Work out the finished part from the listing and answer in its coordinate system (mm). A direction names the side the tool comes from. Coordinates: 2 decimals unless noted, no trailing zeros. Order: outer loops, then holes, each group sorted by start corner. A loop starts at its lowest first (then second) coordinate and runs counter-clockwise, first axis right, second up. Notation, with made-up numbers: (-28.75, 17) -> (-24.75, 17) arc R32 cw to (-24.75, 50) -> close; hole circle Ø7 at (-11, -26.75). An arc over 180 degrees is marked (long way). Use one line per item in the form item = value.
from build123d import *

# Parameters (mm, degrees)
SKETCH1_R                       = 20
BOSS_EXTRUDE1_DEPTH             = 74
SKETCH2_R                       = 2.5
BOSS_EXTRUDE2_DEPTH             = 20
BOSS_EXTRUDE2_DIRECTION_2_REACH = 76
CUT_EXTRUDE1_DEPTH              = 3.81
SKETCH7_R                       = 1.526021313
CUT_EXTRUDE2_DEPTH              = 8.89


with BuildPart() as part:
    # Sketch1 → Boss-Extrude1 (new body)
    with BuildSketch(Plane(origin=(0, 0, 0), x_dir=(0, 0, -1), z_dir=(1, 0, 0))):
        Circle(SKETCH1_R)
    extrude(amount=BOSS_EXTRUDE1_DEPTH)

    # Sketch5 → Cut-Revolve1 (revolve, cut)
    with BuildSketch(Plane(origin=(0, 0, 0), x_dir=(1, 0, 0), z_dir=(0, 1, 0))):
        Polygon((0, 19.337777094), (0.662222906, 20), (0.662222906, 20.176229402), (4.550138216, 20.176229402), (4.550138216, 19.930023338), (4.572872876, 19.930023338), (4.572872876, 20.70759824), (0.489891522, 20.70759824), (-0.879929624, 19.337777094), align=None)
        Polygon((0, 0), (0.645058213, 0), (0.645058213, 3.416287186), (0.081805863, 3.416287186), (0, 3.498093049), (-0.347704824, 3.498093049), (-0.347704824, 0), align=None)
    revolve(axis=Axis((-44.161448521, 0, 0), (1, 0, 0)), mode=Mode.SUBTRACT)

    # Sketch2 → Boss-Extrude2 (add)
    with BuildSketch(Plane.ZY):
        Circle(SKETCH2_R)
    extrude(amount=BOSS_EXTRUDE2_DEPTH)

    # Sketch2 → Boss-Extrude2 direction 2 (add, up to next)
    with BuildSketch(Plane.ZY, mode=Mode.PRIVATE) as boss_extrude2_direction_2_sk1:
        Circle(SKETCH2_R)
    boss_extrude2_direction_2_tool1 = extrude(boss_extrude2_direction_2_sk1.sketch, amount=-BOSS_EXTRUDE2_DIRECTION_2_REACH, mode=Mode.PRIVATE) - part.part
    add(boss_extrude2_direction_2_tool1.solids().sort_by_distance((0, 0, 0))[0])

    # Sketch6 → Cut-Extrude1 (cut)
    with BuildSketch(Plane.ZY):
        with BuildLine():
            Line((-2.93474373, 16.742014233), (-2.93474373, 20.766805635))
            Line((-2.93474373, 20.766805635), (2.93474373, 20.766805635))
            Line((2.93474373, 20.766805635), (2.93474373, 16.742014233))
            ThreePointArc((2.93474373, 16.742014233), (0, 13.807270503), (-2.93474373, 16.742014233))
        make_face()
        with BuildLine():
            Line((20.766805635, -2.93474373), (16.742014233, -2.93474373))
            ThreePointArc((16.742014233, -2.93474373), (13.807270503, 0), (16.742014233, 2.93474373))
            Line((16.742014233, 2.93474373), (20.766805635, 2.93474373))
            Line((20.766805635, 2.93474373), (20.766805635, -2.93474373))
        make_face()
        with BuildLine():
            Line((-2.93474373, -20.766805635), (-2.93474373, -16.742014233))
            ThreePointArc((-2.93474373, -16.742014233), (0, -13.807270503), (2.93474373, -16.742014233))
            Line((2.93474373, -16.742014233), (2.93474373, -20.766805635))
            Line((2.93474373, -20.766805635), (-2.93474373, -20.766805635))
        make_face()
        with BuildLine():
            Line((-20.766805635, 2.93474373), (-16.742014233, 2.93474373))
            ThreePointArc((-16.742014233, 2.93474373), (-13.807270503, 0), (-16.742014233, -2.93474373))
            Line((-16.742014233, -2.93474373), (-20.766805635, -2.93474373))
            Line((-20.766805635, -2.93474373), (-20.766805635, 2.93474373))
        make_face()
    extrude(amount=-CUT_EXTRUDE1_DEPTH, mode=Mode.SUBTRACT)

    # Sketch7 → Cut-Extrude2 (cut)
    with BuildSketch(Plane.ZY):
        with Locations((-3.398071731, 12.681776348)):
            Circle(SKETCH7_R)
        with Locations((9.283704617, 9.283704617)):
            Circle(SKETCH7_R)
        with Locations((12.681776348, -3.398071731)):
            Circle(SKETCH7_R)
        with Locations((3.398071731, -12.681776348)):
            Circle(SKETCH7_R)
        with Locations((-9.283704617, -9.283704617)):
            Circle(SKETCH7_R)
        with Locations((-12.681776348, 3.398071731)):
            Circle(SKETCH7_R)
    extrude(amount=-CUT_EXTRUDE2_DEPTH, mode=Mode.SUBTRACT)


solid = part.part
(1) Which of the six approach directions +Z, -Z, +X, -X, +Y, -Y give full straight-line access (tool end or side, diameter ignored) to faces 1 (the flat face through (2, -2.935, -18)), 2 (the flat face through (2, -2.935, 18)), 3 (the cylindrical face through (4.38, -9.22, -10.81)), 4 (the flat face through (2, -18, -2.935))?
Data:
face_1 = -Z, -X
face_2 = +Z, -X
face_3 = -X
face_4 = -X, -Y
(2) Straight lines are drawn through the part: line 1 along Y through (x, z) = (0.4, 0); line 2 along Z through (x, y) = (20.5, -3); line 3 along X through (y, z) = (-12, 4). For each, find the intervals that lie inside material, in ascending order.
Data:
line_1 = -13.81 to -3.42, -2.5 to 2.5, 3.42 to 13.81
line_2 = -19.77 to 19.77
line_3 = 8.89 to 74
(3) Section C-C on x = 50.5 is taken. Write down the section's boundary in (y, z), plus the area to 3 significant figures.
Data:
outline = circle Ø40 at (0, 0)
area = 1,260 mm²
(4) Each of these flat-tipped pins is pushed along its axis until it touches: P1, Ø1, axis at x = 62, y = 6.5, coming from the -Z side; P2, Ø1.5, axis at x = 50.5, y = -4.5, coming from the -Z side; P3, Ø6, axis at x = 51, y = -2.5, coming from the -Z side; P4, Ø10, axis at y = 9, z = 9.5, coming from the -X side. Where does it stop, or does it pass through?
Data:
P1 = -19.08
P2 = -19.65
P3 = -20
P4 = 0
(5) The mould has two halves that part along Y. Classify faces 5 (the flat face through (2, -18, 2.935)), 6 (the cylindrical face through (1.878, 13.808, 0.065)), 7 (the cylindrical face through (4.383, 3.856, -11.226)): released by +Y, released by -Y, zero draft, split by the parting line, or undercut.
Data:
face_5 = zero draft
face_6 = released by +Y
face_7 = undercut
